Source: CAD feature listing. Evaluate the final solid. Frame: model axes, mm. Face numbers are marked on the shaded views. Round coordinates to 2 decimals unless told otherwise and drop trailing zeros. Order: outer loops, then holes, each group sorted by start corner. A loop starts at its lowest first (then second) coordinate and runs counter-clockwise, first axis right, second up. Notation, with made-up numbers: (13.25, -3) -> (50.25, -3) arc R26 cw to (50.25, 27) -> close; hole circle Ø6 at (70, 81.5). An arc over 180 degrees is marked (long way). Answer as CSV lines item,"result". Start each with the question number.
(1) Section query A-A (y = -35). Output: boundary loops of the cut face in (x, z) (3 decimals), plus the area to 3 significant figures.
(2) Contact query for flat-ended pins moving along their axis: P1, Ø1.1, axis at x = -3, z = 2.5, coming from the -Y side (3 decimals); P2, Ø5, axis at x = 1.5, y = -11.5, coming from the -Z side. Output: stop coordinate, or through.
(3) Section query B-B (z = 3.45). Output: boundary loops of the cut face in (x, y) (3 decimals).
(4) Pull-direction query (Y, two-part tool) for the marked faces 1 and 2; classes: +Y half, -Y half, draft (parallel to the pull), parting line (faces both ways), or undercut.
(5) Section query C-C (x = 0). Output: boundary loops of the cut face in (y, z) (3 decimals).
(6) Section query D-D (y = -10.5). Output: boundary loops of the cut face in (x, z) (3 decimals), plus the area to 3 significant figures.
(7) Line query: line 1 along X through (y, z) = (2.5, 0.5) (3 decimals); line 2 along Y through (x, z) = (-27, 4.35) (3 decimals); line 3 along X through (y, z) = (18, 0.7) (3 decimals). Output: solid intervals per line, ascending. Write a range as from..to.
```python
from build123d import *

# Parameters (mm, degrees)
F0_W     = 69.85
F0_H     = 80.01
F1_DEPTH = 5.08
F3_DEPTH = 1.397
F4_R     = 1
F5_R     = 1
F6_DEPTH = 1.397
F6_TAPER = -8
F7_W     = 12.1412
F7_H     = 22
F8_DEPTH = 3.684
F9_R     = 1.8396307345
F10_R    = 2.0944308897
F11_R    = 21.2450793489


with BuildPart() as f1:
    # F0 (on Top) → F1 (new body)
    with BuildSketch(Plane.XY):
        Rectangle(F0_W, F0_H)
    extrude(amount=F1_DEPTH)

    # F2 (on Top) → F3 (cut)
    with BuildSketch(Plane.XY):
        with BuildLine():
            ThreePointArc((6.0706, 15.0231522067), (0, 21.0937522067), (-6.0706, 15.0231522067))
            Line((-6.0706, 15.0231522067), (-6.0706, -3.937))
            Line((-6.0706, -3.937), (-6.0706, -8.7576295534))
            ThreePointArc((-6.0706, -8.7576295534), (-4.662, -10.9752828266), (-6.0706, -13.1929360997))
            Line((-6.0706, -13.1929360997), (-6.0706, -17.907))
            Line((-6.0706, -17.907), (-6.0706, -40.7645274005))
            Line((-6.0706, -40.7645274005), (6.0706, -40.7645274005))
            Line((6.0706, -40.7645274005), (6.0706, -13.1929360997))
            ThreePointArc((6.0706, -13.1929360997), (4.662, -10.9752828266), (6.0706, -8.7576295534))
            Line((6.0706, -8.7576295534), (6.0706, -3.937))
            Line((6.0706, -3.937), (6.0706, 15.0231522067))
        make_face()
    extrude(amount=F3_DEPTH, mode=Mode.SUBTRACT)

    # F4
    f4_edges = [f1.edges().sort_by_distance(p)[0] for p in [
        (-6.0706, -13.192936, 0.6985),
        (6.0706, -13.192936, 0.6985),
    ]]
    fillet(f4_edges, radius=F4_R)

    # F5 (on face) → F6 (join, through all)
    with BuildSketch(Plane(origin=(0, 0, 0), x_dir=(1, 0, 0), z_dir=(0, 0, -1))):
        with Locations((0, -15.171)):
            Circle(F5_R)
    extrude(amount=-F6_DEPTH, taper=F6_TAPER)

    # F7 (on face) → F8 (cut, through all)
    with BuildSketch(Plane(origin=(0, 0, 1.397), x_dir=(1, 0, 0), z_dir=(0, 0, -1))):
        with Locations((0, 29.005)):
            Rectangle(F7_W, F7_H)
    extrude(amount=-F8_DEPTH, mode=Mode.SUBTRACT)

    # F9
    f9_edges = [f1.edges().sort_by_distance(p)[0] for p in [
        (34.925, -40.005, 2.54),
        (-34.925, -40.005, 2.54),
        (-34.925, 40.005, 2.54),
        (34.925, 40.005, 2.54),
    ]]
    fillet(f9_edges, radius=F9_R)

    # F10
    f10_edges = [f1.edges().sort_by_distance(p)[0] for p in [
        (6.0706, -8.75763, 0.6985),
        (-6.0706, -8.75763, 0.6985),
    ]]
    fillet(f10_edges, radius=F10_R)

    # F11
    f11_edges = [f1.edges().sort_by_distance(p)[0] for p in [
        (6.0706, -40.005, 2.54),
        (-6.0706, -40.005, 2.54),
    ]]
    fillet(f11_edges, radius=F11_R)


solid = f1.part
```
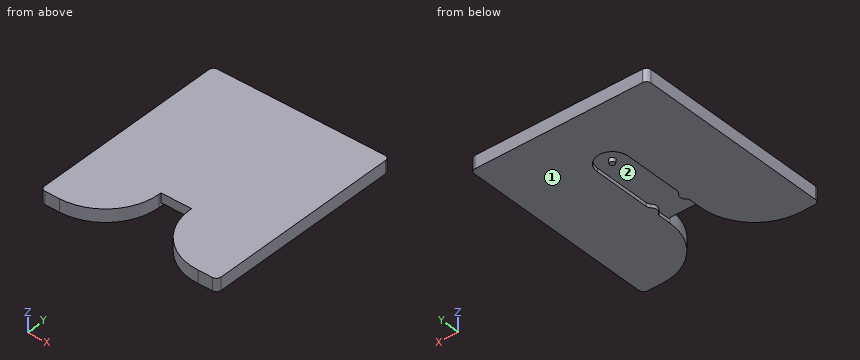
Answer block:
1,outline,"(-34.925, 0) -> (-13.618, 0) -> (-13.618, 5.08) -> (-34.925, 5.08) -> close; (13.618, 0) -> (34.925, 0) -> (34.925, 5.08) -> (13.618, 5.08) -> close"
1,area,"216 mm2"
2,P1,"y = -18.005"
2,P2,"z = 1.4"
3,outline,"(-34.925, -38.165) arc R1.84 ccw to (-33.085, -40.005) -> (-27.316, -40.005) arc R21.245 ccw to (-6.071, -18.76) -> (-6.071, -18.005) -> (6.071, -18.005) -> (6.071, -18.76) arc R21.245 ccw to (27.316, -40.005) -> (33.085, -40.005) arc R1.84 ccw to (34.925, -38.165) -> (34.925, 38.165) arc R1.84 ccw to (33.085, 40.005) -> (-33.085, 40.005) arc R1.84 ccw to (-34.925, 38.165) -> close"
4,face 1,"draft"
4,face 2,"undercut"
5,outline,"(-18.005, 1.397) -> (13.975, 1.397) -> (14.171, 0) -> (16.171, 0) -> (16.367, 1.397) -> (21.094, 1.397) -> (21.094, 0) -> (40.005, 0) -> (40.005, 5.08) -> (-18.005, 5.08) -> close"
6,outline,"(-34.925, 0) -> (-4.709, 0) -> (-4.709, 1.397) -> (4.709, 1.397) -> (4.709, 0) -> (34.925, 0) -> (34.925, 5.08) -> (-34.925, 5.08) -> close"
6,area,"342 mm2"
7,line 1,"-34.925..-6.071, 6.071..34.925"
7,line 2,"-40.003..40.005"
7,line 3,"-34.925..-5.291, 5.291..34.925"
